```python
from build123d import *

# Parameters (mm, degrees)
F0_W     = 88.9
F0_H     = 63.5
F1_DEPTH = 63.5
F3_T     = -2.54
F2_R     = 10.16
F4_DEPTH = 25.4


with BuildPart() as f1:
    # F0 (on Top) → F1 (new body)
    with BuildSketch(Plane.XY):
        with Locations((10.68233, 16.748335)):
            Rectangle(F0_W, F0_H)
    extrude(amount=F1_DEPTH)

    # F3
    f3_openings = [f1.faces().sort_by_distance(p)[0] for p in [
        (-33.76767, 16.748335, 31.75),
    ]]
    offset(amount=F3_T, openings=f3_openings)

    # F2 (on face) → F4 (cut)
    with BuildSketch(Plane.YZ.offset(55.13233)):
        with Locations((-2.301665, 27.94)):
            Circle(F2_R)
        with Locations((35.798335, 27.94)):
            Circle(F2_R)
    extrude(amount=-F4_DEPTH, mode=Mode.SUBTRACT)


solid = f1.part
```
Design review of the part built by this model. Coordinates are the model's own, in mm. A direction names the side the tool comes from. Coordinates: 2 decimals unless noted, no trailing zeros. Order: outer loops, then holes, each group sorted by start corner. A loop starts at its lowest first (then second) coordinate and runs counter-clockwise, first axis right, second up. Notation, with made-up numbers: M 1,27 L 10,27 A23 ccw 10,64 Z; hole C 26.25,79.25 d7. An arc over 180 degrees is marked long. Answer as a JSON object with one key per item and string values. Group by question number.
1) Wall thickness on L1, parallel to Y at x = 47, z = 37.5; L2, parallel to Z at x = 51.5, y = -4.5; L3, parallel to Y at x = 53, z = 27: over which ranges is each line inside the solid? List them lowest first.
2) Mouldability with a two-part tool opening along Y and no side actions: class faces 1 (the flat face through (9, 17, 60.96)), 2 (the flat face through (-33.768, 14, 62)), 3 (the flat face through (10, 48.498, 31)), 4 (the flat face through (10, -15.002, 31)) as pulls with the +Y half, pulls with the -Y half, needs draft (parallel to the pull), parting line crosses it, or undercut.
3) Add section D-D, the plane z = 59. Write out the cut boundary in (x, y).
4) Tool access review of faces 5 (the flat face through (9, 45.958, 31)), 6 (the flat face through (55.132, 16, 31)): name each direction out of +Z, -Z, +X, -X, +Y, -Y from which nothing blocks a thin tool from reaching the whole face with its end or side.
5) Add section B-B, the plane y = -4.5. Write out the cut boundary in (x, z).
6) Add section C-C, the plane z = 23. Write out the cut boundary in (x, y), then the cut area to 3 significant figures.
7) For pin 1 (1.5 mm diameter, centred on x = -14.5, y = 18.5, fed in from -Z); pin 2 (12 mm diameter, centred on y = 35.8, z = 27.94, fed in from -X), all flat-tipped, find the tip position at first contact; note any pin that passes through.
8) Add section A-A, the plane x = 15.5. Write out the cut boundary in (y, z).
Computed values:
{
 "1": {"L1": "y = -15 to -12.46, 45.96 to 48.5", "L2": "z = 0 to 2.54, 60.96 to 63.5", "L3": "y = -15 to -12.42, 7.81 to 25.68, 45.91 to 48.5"},
 "2": {"face 1": "undercut", "face 2": "needs draft", "face 3": "pulls with the +Y half", "face 4": "pulls with the -Y half"},
 "3": {"outline": "M -33.77,-15 L 55.13,-15 L 55.13,48.5 L -33.77,48.5 L -33.77,45.96 L 52.59,45.96 L 52.59,-12.46 L -33.77,-12.46 Z"},
 "4": {"face 5": "-X", "face 6": "+Z, -Z, +X, +Y, -Y"},
 "5": {"outline": "M -33.77,0 L 55.13,0 L 55.13,18.02 L 52.59,18.02 L 52.59,2.54 L -33.77,2.54 Z; M -33.77,60.96 L 52.59,60.96 L 52.59,37.86 L 55.13,37.86 L 55.13,63.5 L -33.77,63.5 Z"},
 "6": {"outline": "M -33.77,-15 L 55.13,-15 L 55.13,-11.18 L 52.59,-11.18 L 52.59,-12.46 L -33.77,-12.46 Z; M -33.77,45.96 L 52.59,45.96 L 52.59,44.68 L 55.13,44.68 L 55.13,48.5 L -33.77,48.5 Z; M 52.59,6.58 L 55.13,6.58 L 55.13,26.92 L 52.59,26.92 Z", "area": "510 mm^2"},
 "7": {"pin 1": "stops at z = 0", "pin 2": "passes through"},
 "8": {"outline": "M -15,0 L 48.5,0 L 48.5,63.5 L -15,63.5 Z; hole M -12.46,2.54 L 45.96,2.54 L 45.96,60.96 L -12.46,60.96 Z"}
}
